The listing builds one solid part. Answer for the finished solid, in the listing's coordinates (mm). A direction names the side the tool comes from. Round coordinates to 2 decimals unless told otherwise and drop trailing zeros. Write each loop counter-clockwise with the first axis right and the second up, starting at its lowest first coordinate (ties: lowest second). Pieces come first, ordered by that corner, then holes.
from build123d import *

# Parameters (mm, degrees)
F5_DEPTH = 1
F7_DEPTH = 1
F9_DEPTH = 1


with BuildPart() as f3:
    # F0 (on Top) → F3 section 0
    with BuildSketch(Plane.XY, mode=Mode.PRIVATE) as f3_s0:
        Polygon((-14.4337567297, 25), (-14.4337567297, -25), (28.8675134595, 0), align=None)
    loft([f3_s0.sketch, Vertex(0, 0, 35)])

    # F4 (on face) → F5 (cut)
    with BuildSketch(Plane(origin=(-12.3358269725, 0, 5.0872093023), x_dir=(0, -1, 0), z_dir=(-0.9244734516, 0, 0.3812464258))):
        Polygon((-2, -0.5028181645), (0, -0.5028181645), (0, 9.4971818355), (0, 11.4971818355), (0, 17.4971818355), (0, 19.4971818355), (-2, 19.4971818355), align=None)
        with BuildLine():
            Line((0, 11.4971818355), (0, 9.4971818355))
            ThreePointArc((0, 9.4971818355), (5, 14.4971818355), (0, 19.4971818355))
            Line((0, 19.4971818355), (0, 17.4971818355))
            ThreePointArc((0, 17.4971818355), (3, 14.4971818355), (0, 11.4971818355))
        make_face()
    extrude(amount=-F5_DEPTH, mode=Mode.SUBTRACT)

    # F6 (on face) → F7 (cut)
    with BuildSketch(Plane(origin=(6.1679134863, -10.6831395349, 5.0872093023), x_dir=(0.8867565671, 0.4173352901, -0.1987310905), z_dir=(0.4622367258, -0.8006174942, 0.3812464258))):
        with BuildLine():
            Line((-0.7380038788, 19.4712978038), (-2.691246597, 19.0413642234))
            ThreePointArc((-2.691246597, 19.0413642234), (-10.3077922864, 7.1254827301), (1.6080892069, -0.4910629592))
            Line((1.6080892069, -0.4910629592), (3.5613319251, -0.0611293789))
            Line((3.5613319251, -0.0611293789), (3.1313983448, 1.8921133394))
            Line((3.1313983448, 1.8921133394), (1.1781556265, 1.462179759))
            ThreePointArc((1.1781556265, 1.462179759), (-8.3545495681, 7.5554163105), (-2.2613130166, 17.0881215051))
            Line((-2.2613130166, 17.0881215051), (-0.3080702984, 17.5180550855))
            Line((-0.3080702984, 17.5180550855), (-0.7380038788, 19.4712978038))
        make_face()
    extrude(amount=-F7_DEPTH, mode=Mode.SUBTRACT)

    # F8 (on face) → F9 (cut)
    with BuildSketch(Plane(origin=(6.1679134863, 10.6831395349, 5.0872093023), x_dir=(-0.8867565671, 0.4173352901, 0.1987310905), z_dir=(0.4622367258, 0.8006174942, 0.3812464258))):
        Polygon((2.3919107931, -0.2709502327), (3.3919107931, -0.4910629592), (3.3919107931, 14.4979807209), (3.0442146526, 14.5745130664), (-3.9632350967, 2.4372540691), (-3.9632350967, 16.4866717508), (-4.1080892069, 16.518555984), (-11.6080892069, 3.5281749272), (-10.5972096929, 3.2790696058), (-4.9632350967, 13.037399855), (-4.9632350967, 1.6334285103), (-4.1782018869, 1.46063271), (-3.4632453686, 1.3032616814), (2.3919107931, 11.4446896398), align=None)
        with BuildLine():
            ThreePointArc((5.1544700324, -0.6785410767), (9.4095342954, 1.5116065738), (8.0476246724, 6.0993642823))
            ThreePointArc((8.0476246724, 6.0993642823), (11.5155654495, 9.8960628609), (8.3789718853, 13.9707793103))
            Line((8.3789718853, 13.9707793103), (7.4023505262, 14.1857461004))
            Line((7.4023505262, 14.1857461004), (4.1778486732, -0.4635742865))
            Line((4.1778486732, -0.4635742865), (5.1544700324, -0.6785410767))
        make_face()
        with BuildLine():
            ThreePointArc((6.5517541686, 5.6694977576), (8.6463042332, 2.392630347), (5.3694368226, 0.2980802824))
            Line((5.3694368226, 0.2980802824), (5.9605954956, 2.98378902))
            Line((5.9605954956, 2.98378902), (6.0680788907, 3.4720996996))
            Line((6.0680788907, 3.4720996996), (6.5517541686, 5.6694977576))
        make_face(mode=Mode.SUBTRACT)
        with BuildLine():
            ThreePointArc((8.0476246724, 6.0993642823), (7.3508737117, 6.0678331487), (6.6592375637, 6.1578084372))
            Line((6.6592375637, 6.1578084372), (6.7667209588, 6.6461191168))
            ThreePointArc((6.7667209588, 6.6461191168), (7.4327779419, 6.4327278198), (8.0476246724, 6.0993642823))
        make_face(mode=Mode.SUBTRACT)
        with BuildLine():
            ThreePointArc((8.1640050951, 12.9941579511), (10.4489688019, 9.4193935031), (6.8742043539, 7.1344297963))
            Line((6.8742043539, 7.1344297963), (7.4116213294, 9.5759831942))
            Line((7.4116213294, 9.5759831942), (7.5191047245, 10.0642938737))
            Line((7.5191047245, 10.0642938737), (8.1640050951, 12.9941579511))
        make_face(mode=Mode.SUBTRACT)
        with BuildLine():
            Line((6.7667209588, 6.6461191168), (6.6592375637, 6.1578084372))
            ThreePointArc((6.6592375637, 6.1578084372), (7.3508737117, 6.0678331487), (8.0476246724, 6.0993642823))
            ThreePointArc((8.0476246724, 6.0993642823), (7.4327779419, 6.4327278198), (6.7667209588, 6.6461191168))
        make_face()
    extrude(amount=-F9_DEPTH, mode=Mode.SUBTRACT)


solid = f3.part
1. For a pull along X with two mould halves and no side action, classify faces 4 (the face through (-1.208, 10.207, 12.408)), 5 (the face through (3, 0, 0)), 6 (the face through (-10.323, 5.906, 9.967)), 7 (the face through (4.663, 7.376, 13.856)) as released by +X, released by -X, zero draft, split by the parting line, or undercut.
Geometry says:
face 4: undercut
face 5: zero draft
face 6: released by -X
face 7: released by +X
2. Section C-C on x = 26.5 is taken. Determine the outline of the cut face in (y, z).
Geometry says:
outline: (-1.37, 0) - (1.37, 0) - (0, 2.87) - close
3. Given pin 1 (12 mm diameter, centred on y = 9, z = 28.5, fed in from -X); pin 2 (12 mm diameter, centred on x = 15.5, z = 22, fed in from +Y); pin 3 (2 mm diameter, centred on y = -15, z = 13.5, fed in from +X), each flat-ended and moving along its own axis, determine where each tip first touches the part or whether it passes through.
Geometry says:
pin 1: stops at x = -5.15
pin 2: stops at y = 1.73
pin 3: stops at x = -6.33
4. A tool of negligible diameter and unlimited length cuts with its end or side. For faces 1 (the face through (2.932, 8.738, 11.802)), 2 (the face through (12.874, 3.547, 10.649)), 3 (the face through (4.432, -2.718, 22.626)), from which of +Z, -Z, +X, -X, +Y, -Y can it reach the whole face along a straight path? Write none if from no direction.
Geometry says:
face 1: none
face 2: +Z
face 3: -Y
5. Section A-A on x = 14 is taken. Determine the outline of the cut face in (y, z).
Geometry says:
outline: (-8.58, 0) - (8.58, 0) - (4.27, 9.05) - (3.64, 7.75) - (2.78, 9.56) - (3.41, 10.86) - (0, 18.03) - close
6. Section B-B on z = 25 is taken. Determine the outline of the cut face in (x, y).
Geometry says:
outline: (-4.12, -7.14) - (8.25, 0) - (-4.12, 7.14) - close
7. Straight lines are drawn through the part: line 1 along Z through (x, y) = (-7, 18.5); line 2 along Z through (x, y) = (11.5, 5.5); line 3 along Y through (x, z) = (1, 26.5). For each, find the intervals that lie inside material, in ascending order.
Geometry says:
line 1: z = 0 to 4.64
line 2: z = 0 to 9.51
line 3: y = -3.47 to 3.47
